Here's how the part is built. I have some questions about the finished solid (model axes, mm). A direction names the side the tool comes from. Give positions to 0.01 mm unless a question says otherwise; leave off trailing zeros. Loops run counter-clockwise (first coordinate to the right, second up) from the corner with the lowest first, then second, coordinate; pieces in that order, holes last.
Q1. If we section it at A-A (z = 12.5): Please give me the cut outline in (x, y).
Q2. We'd pull the mould along Y, two halves only. Please class faces 1 (the face through (-19, 1, 3)), 2 (the face through (-8, -8.75, 15)), 3 (the face through (-8, -57, 16)): +Y half, -Y half, draft (parallel to the pull), parting line (faces both ways), or undercut.
Q3. If we section it at D-D (y = -4.5): Give the number of separate pieces and of enclosed holes in the cut face, plus the area to 3 significant figures.
Q4. For faces 4 (the face through (-10.5, -24.1, 4.6)), 5 (the face through (-8, -49.25, 15)), 6 (the face through (-13, -19, 28.5)), 7 (the face through (5, -19, 28.75)), 8 (the face through (5, -19, 1.25)), which set-ups out of +Z, -Z, +X, -X, +Y, -Y let a thin tool reach every point of the face, with its end or its side?
Q5. If we section it at C-C (y = -53.5): Please give me the cut outline in (x, z) (3 decimals).
Q6. I need wall thicknesses on line 1 (Z direction, x = -8, y = -53); line 2 (Z direction, x = 17.5, y = 2.1); line 3 (Z direction, x = 9.5, y = -3.5). Which ranges of each line are inside material? Lowest first, please.
Q7. If we section it at B-B (x = -17.5): Please give me the cut outline in (y, z).
Q8. Will these pins go through, and if not, where does the flat tip stop? P1, Ø1, axis at x = 15.5, y = -7, coming from the -Z side; P2, Ø2.5, axis at x = 17.5, z = 31, coming from the +Y side; P3, Ø3.5, axis at y = -53.5, z = 10, coming from the +X side; P4, Ø6, axis at x = -5, y = -42.5, coming from the -Z side.
from build123d import *

# Parameters (mm, degrees)
F0_R       = 1.5
F1_DEPTH   = 3
F3_DEPTH   = 57
F4_R       = 1.625
F4_W       = 40.5
F4_H       = 20
F5_DEPTH   = 33.001
F2_W       = 28.2747811079
F2_H       = 3
F6_DEPTH   = 50
F7_SIZE2   = 50
F7_SIZE    = 28
F7_2_SIZE2 = 50
F7_2_SIZE  = 28
F8_SIZE2   = 55
F8_SIZE    = 5
F9_R       = 10.70545329
F10_W      = 6
F10_H      = 3
F11_DEPTH  = 50
F12_SIZE2  = 49.99999
F12_SIZE   = 5.99999


# Not quite as in the source:
# - a fillet or chamfer is up to 0.001 mm smaller than in the source, because OpenCascade refuses the exact size


with BuildPart() as f1:
    # F0 (on Front) → F1 (new body)
    with BuildSketch(Plane.XZ):
        Polygon((-22.5, 23), (-22.5, 0), (22.5, 0), (22.5, 32), (19.5, 35), (-10.5, 35), align=None)
        with Locations((-17.5, 3)):
            Circle(F0_R, mode=Mode.SUBTRACT)
        with Locations((17.5, 31)):
            Circle(F0_R, mode=Mode.SUBTRACT)
    extrude(amount=-F1_DEPTH)

    # F2 (on face) → F3 (join)
    with BuildSketch(Plane.XZ):
        Polygon((-5.7747811079, 35), (-10.5, 35), (-10.5, 0), (-5.7747811079, 0), (-5.7747811079, 1.25), (-5.7747811079, 4.25), (-5.7747811079, 25.75), (-5.7747811079, 28.75), align=None)
    extrude(amount=F3_DEPTH)

    # F4 (on face) → F5 (cut, through all)
    with BuildSketch(Plane(origin=(-10.5, 0, 0), x_dir=(0, -1, 0), z_dir=(-1, 0, 0))):
        with Locations((4.5, 20)):
            Circle(F4_R)
        with Locations((4.5, 10)):
            Circle(F4_R)
        with Locations((29, 15)):
            Rectangle(F4_W, F4_H)
        with Locations((53.5, 20)):
            Circle(F4_R)
        with Locations((53.5, 10)):
            Circle(F4_R)
    extrude(amount=-F5_DEPTH, mode=Mode.SUBTRACT)

    # F2 (on face) → F6 (join)
    with BuildSketch(Plane.XZ):
        with Locations((8.362609446, 27.25)):
            Rectangle(F2_W, F2_H)
        with Locations((8.362609446, 2.75)):
            Rectangle(F2_W, F2_H)
    extrude(amount=F6_DEPTH)

    # F7
    f7_edges = [f1.edges().sort_by_distance(p)[0] for p in [
        (22.5, -50, 27.25),
    ]]
    f7_side = f1.faces().sort_by_distance((8.362609, -50, 27.25))[0]
    chamfer(f7_edges, length=F7_SIZE, length2=F7_SIZE2, reference=f7_side)

    # F7#2
    f7_2_edges = [f1.edges().sort_by_distance(p)[0] for p in [
        (22.5, -50, 2.75),
    ]]
    f7_2_side = f1.faces().sort_by_distance((8.362609, -50, 2.75))[0]
    chamfer(f7_2_edges, length=F7_2_SIZE, length2=F7_2_SIZE2, reference=f7_2_side)

    # F8
    f8_edges = [f1.edges().sort_by_distance(p)[0] for p in [
        (-8.137391, -57, 35),
    ]]
    chamfer(f8_edges, length=F8_SIZE, length2=F8_SIZE2)

    # F9
    f9_edges = [f1.edges().sort_by_distance(p)[0] for p in [
        (-8.137391, -57, 30),
        (-8.137391, -57, 0),
    ]]
    fillet(f9_edges, radius=F9_R)

    # F10 (on face) → F11 (join)
    with BuildSketch(Plane.XZ):
        with Locations((-13.5, 27)):
            Rectangle(F10_W, F10_H)
    extrude(amount=F11_DEPTH)

    # F12 (size 6 and 50 in the source; OpenCascade refuses exactly that, so slightly less here)
    f12_edges = [f1.edges().sort_by_distance(p)[0] for p in [
        (-16.5, -50, 27),
    ]]
    f12_side = f1.faces().sort_by_distance((-13.5, -50, 27))[0]
    chamfer(f12_edges, length=F12_SIZE, length2=F12_SIZE2, reference=f12_side)


solid = f1.part
Check sheet entries:
1. outline: (-22.5, 0) - (-10.5, 0) - (-10.5, -8.75) - (-5.77, -8.75) - (-5.77, 0) - (22.5, 0) - (22.5, 3) - (-22.5, 3) - close; (-10.5, -57) - (-5.77, -57) - (-5.77, -49.25) - (-10.5, -49.25) - close
2. face 1: draft
2. face 2: undercut
2. face 3: -Y half
3. separate pieces: 3
3. enclosed holes: 0
3. area: 305 mm2
4. face 4: -X, -Y
4. face 5: +X, -X
4. face 6: +Z, -X, -Y
4. face 7: +Z, +X, -Y
4. face 8: -Z, +X, -Y
5. outline: (-10.5, 2.788) - (-5.775, 2.788) - (-5.775, 8.375) - (-10.5, 8.375) - close; (-10.5, 11.625) - (-5.775, 11.625) - (-5.775, 18.375) - (-10.5, 18.375) - close; (-10.5, 21.625) - (-5.775, 21.625) - (-5.775, 28.141) - (-10.5, 28.141) - close
6. line 1: z = 2.36 to 8.45, 11.55 to 18.45, 21.55 to 28.57
6. line 2: z = 0 to 29.5, 32.5 to 35
6. line 3: z = 1.25 to 4.25, 25.75 to 28.75
7. outline: (0, 0) - (3, 0) - (3, 1.5) - (0, 1.5) - close; (0, 4.5) - (3, 4.5) - (3, 28) - (0, 28) - close
8. P1: stops at z = 1.25
8. P2: passes through
8. P3: stops at x = -5.77
8. P4: stops at z = 0
